from build123d import *

# Parameters (mm, degrees)
F0_W     = 50.8
F0_H     = 85.725
F1_DEPTH = 3.175
F2_W     = 3.175
F2_H     = 42.8625
F3_DEPTH = 3.175


with BuildPart() as f1:
    # F0 (on Front) → F1 (new body)
    with BuildSketch(Plane.XZ):
        with Locations((0, 42.8625)):
            Rectangle(F0_W, F0_H)
    extrude(amount=F1_DEPTH)

    # F2 (on face) → F3 (cut)
    with BuildSketch(Plane.XZ.offset(3.175)):
        with Locations((0, 21.43125)):
            Rectangle(F2_W, F2_H)
    extrude(amount=-F3_DEPTH, mode=Mode.SUBTRACT)


with BuildPart() as f4_1:
    # F4: copy of F1
    add(f1.part)


solid = f1.part
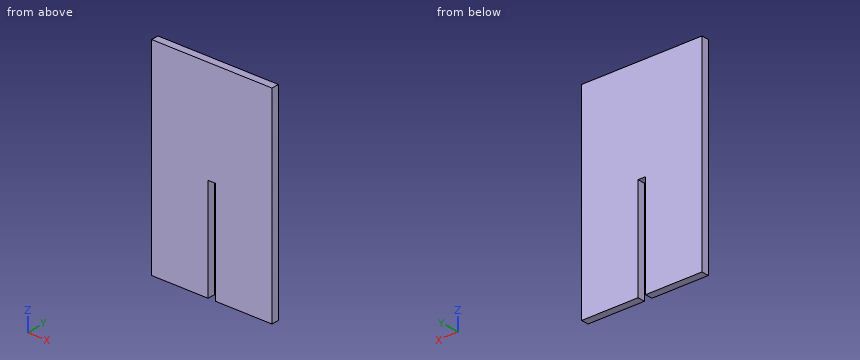
Can you work these out from the model? Positions are in its coordinate system, mm. Round coordinates to 2 decimals unless told otherwise and drop trailing zeros. Write each loop counter-clockwise with the first axis right and the second up, starting at its lowest first coordinate (ties: lowest second). Pieces come first, ordered by that corner, then holes. Notation, with made-up numbers: (42, 84.5) -> (87, 84.5) arc R4 cw to (87, 88.5) -> close; hole circle Ø7 at (55, -19.5). An arc over 180 degrees is marked (long way). One line per question, with ' | ' between items. Start each with the question number.
1) Suppose I cut it at A-A on z = 14. Write out the boundary of the cut face in (x, y) (1 decimal), then the cut area to 3 significant figures.
2) I need wall thicknesses on line 1 (X direction, y = -0.2, z = 15.5); line 2 (Z direction, x = 0, y = -1.4) (1 decimal). Which ranges of each line are inside material? Lowest first, please. Write a range as [from, to].
3) Suppose I cut it at B-B on y = -2.5. Write out the boundary of the cut face in (x, z) (1 decimal).
Return value:
1) outline: (-25.4, -3.2) -> (-1.6, -3.2) -> (-1.6, 0) -> (-25.4, 0) -> close; (1.6, -3.2) -> (25.4, -3.2) -> (25.4, 0) -> (1.6, 0) -> close | area: 151 mm2
2) line 1: x = [-25.4, -1.59], [1.59, 25.4] | line 2: z = [42.9, 85.7]
3) outline: (-25.4, 0) -> (-1.6, 0) -> (-1.6, 42.9) -> (1.6, 42.9) -> (1.6, 0) -> (25.4, 0) -> (25.4, 85.7) -> (-25.4, 85.7) -> close
